Geometry: final body of the model. Coordinates: model frame, mm. A direction names the side the tool comes from. Round coordinates to 2 decimals unless told otherwise and drop trailing zeros. Loops run counter-clockwise (first coordinate to the right, second up) from the corner with the lowest first, then second, coordinate; pieces in that order, holes last. Notation, with made-up numbers: M 4.5,-40 L 18.5,-40 A4 cw 18.5,-35 Z; hole C 43.25,56 d3. An arc over 180 degrees is marked long. Return JSON: item names as keys, results as strings.
from build123d import *


with BuildPart() as part:
    # Sketch1 → Revolve1 (revolve)
    with BuildSketch(Plane.XY, mode=Mode.PRIVATE) as revolve1_sk:
        with BuildLine():
            Line((0, -4.7625), (0, 0))
            Line((0, 0), (50.8, 0))
            ThreePointArc((50.8, 0), (50.642418278, -0.418684593), (50.247884132, -0.629567487))
            Line((50.247884132, -0.629567487), (43.453994693, -1.524))
            Line((43.453994693, -1.524), (29.628156352, -1.524))
            Line((29.628156352, -1.524), (27.94, -1.74625))
            Line((27.94, -1.74625), (5.08, -1.74625))
            Line((5.08, -1.74625), (3.048, -2.54))
            Line((3.048, -2.54), (0.8255, -4.7625))
            Line((0.8255, -4.7625), (0, -4.7625))
        make_face()
    revolve(revolve1_sk.sketch.rotate(Axis((0, 0, 0), (1, 0, 0)), 270), axis=Axis((0, 0, 0), (1, 0, 0)))


solid = part.part
Q1. Material intervals for L1, parallel to Y at x = 44, z = -1; L2, parallel to X at y = -2.5, z = -1.75; L3, parallel to Z at x = 28, y = -0.25, sorted ascending.
Determined:
{"L1": "y = -1.05 to 1.05", "L2": "x = 0 to 2.54", "L3": "z = -1.72 to 1.72"}
Q2. Section query D-D (x = 40). Output: boundary loops of the cut face in (y, z), plus the area to 3 significant figures.
Determined:
{"outline": "C 0,0 d3.05", "area": "7.30 mm^2"}
Q3. Reachability of faces 1 (the cylindrical face through (36.444, -1.285, 0.819)), 2 (the cylindrical face through (0.41, 2.9, -3.78)) from +Z, -Z, +X, -X, +Y, -Y: full face, straight path, thin tool, end or side. Return the list, or none.
Determined:
{"face 1": "+X", "face 2": "+X, -X"}
Q4. Section query A-A (y = 0). Output: boundary loops of the cut face in (x, z) (1 decimal).
Determined:
{"outline": "M 0,-4.8 L 0.8,-4.8 L 3,-2.5 L 5.1,-1.7 L 27.9,-1.7 L 29.6,-1.5 L 43.5,-1.5 L 50.2,-0.6 A0.6 ccw 50.2,0.6 L 43.5,1.5 L 29.6,1.5 L 27.9,1.7 L 5.1,1.7 L 3,2.5 L 0.8,4.8 L 0,4.8 Z"}
Q5. Section query C-C (x = 16). Output: boundary loops of the cut face in (y, z), plus the area to 3 significant figures.
Determined:
{"outline": "C 0,0 d3.49", "area": "9.58 mm^2"}
Q6. Pin query (flat end, axial travel): pin 1 (1 mm diameter, centred on x = 32, z = 1, fed in from +Y); pin 2 (1 mm diameter, centred on x = 11.5, z = -2, fed in from -Y). Return the tip coordinate at first contact, or that it passes through.
Determined:
{"pin 1": "stops at y = 1.44", "pin 2": "stops at y = -0.89"}
